Read the model definition and answer for the solid it produces. Units are mm, in the model's axes. Face numbers are marked on the shaded views. A direction names the side the tool comes from. Coordinates: 2 decimals unless noted, no trailing zeros. Write each loop counter-clockwise with the first axis right and the second up, starting at its lowest first coordinate (ties: lowest second). Pieces come first, ordered by that corner, then holes. Notation, with made-up numbers: (48.25, 45.25) -> (81.25, 45.25) arc R31 cw to (81.25, 70.25) -> close; hole circle Ø5 at (73, 83). An arc over 180 degrees is marked (long way). Answer as a JSON object with one key per item and string values. Group by question number.
(1) Find section A-A (z = 28.5). Give the vertices of the cut face in (x, y), then the cut area to 3 significant figures.
(2) Straight lines are drawn through the part: L1, parallel to Z at x = -12, y = -4; L2, parallel to Z at x = 17, y = -2.25; L3, parallel to X at y = 4.75, z = 33. For each, find the intervals that lie inside material, in ascending order.
(3) Find section C-C (x = -38). Give the vertices of the cut face in (y, z), then the cut area to 3 significant figures.
(4) Find section B-B (z = 6.5). Give the vertices of the cut face in (x, y).
(5) Which of the six approach directions +Z, -Z, +X, -X, +Y, -Y give full straight-line access (tool end or side, diameter ignored) to the marked faces 1 and 2?
(6) For a pull along X with two mould halves and no side action, classify the marked faces 3, 4, 5 and 6 as +X half, -X half, draft (parallel to the pull), parting line (faces both ways), or undercut.
(7) Flat-ended cylindrical pins translate along their axes: P1, Ø4, axis at x = -156.5, y = -1.5, coming from the +Z side; P2, Ø6, axis at y = 3.5, z = 30, coming from the -X side; P3, Ø6, axis at y = -6.5, z = 22, coming from the +X side. Find the tip coordinate at first contact, or state that the pin passes through.
(8) Find section D-D (y = -2.25). Give the vertices of the cut face in (x, z).
from build123d import *

# Parameters (mm, degrees)
F1_DEPTH = 35
F3_DEPTH = 10
F5_DEPTH = 12
F6_DEPTH = 12


with BuildPart() as f1:
    # F0 (on Top) → F1 (new body)
    with BuildSketch(Plane.XY):
        with BuildLine():
            Line((-62.8165142711, -9.8129920568), (57.1834857289, -9.8129920568))
            Line((57.1834857289, -9.8129920568), (92.1834857289, -4.8627543336))
            Line((92.1834857289, -4.8627543336), (92.8836937573, -4.7637201565))
            ThreePointArc((92.8836937573, -4.7637201565), (95.958471831, -3.0916320079), (97.1834857289, 0.1870079432))
            ThreePointArc((97.1834857289, 0.1870079432), (95.958471831, 3.4656478942), (92.8836937573, 5.1377360428))
            Line((92.8836937573, 5.1377360428), (57.1834857289, 10.1870079432))
            Line((57.1834857289, 10.1870079432), (-62.8165142711, 10.1870079432))
            Line((-62.8165142711, 10.1870079432), (-162.8165142711, 5.1870079432))
            ThreePointArc((-162.8165142711, 5.1870079432), (-167.8165142711, 0.1870079432), (-162.8165142711, -4.8129920568))
            Line((-162.8165142711, -4.8129920568), (-62.8165142711, -9.8129920568))
        make_face()
    extrude(amount=F1_DEPTH)

    # F2 (on face) → F3 (join)
    with BuildSketch(Plane.XY.offset(35)):
        with BuildLine():
            Line((57.1834857289, 10.1870079432), (27.1834857289, 10.1870079432))
            Line((27.1834857289, 10.1870079432), (27.1834857289, -9.8129920568))
            Line((27.1834857289, -9.8129920568), (57.1834857289, -9.8129920568))
            Line((57.1834857289, -9.8129920568), (92.8836937573, -4.7637201565))
            ThreePointArc((92.8836937573, -4.7637201565), (97.1834857289, 0.1870079432), (92.8836937573, 5.1377360428))
            Line((92.8836937573, 5.1377360428), (57.1834857289, 10.1870079432))
        make_face()
    extrude(amount=F3_DEPTH)

    # F4 (on face) → F5 (cut)
    with BuildSketch(Plane.XY.offset(35)):
        Polygon((2.1834857289, -9.8129920568), (2.1834857289, 10.1870079432), (-62.8165142711, 10.1870079432), (-67.8165142711, 9.9370079432), (-67.8165142711, -9.5629920568), (-62.8165142711, -9.8129920568), align=None)
    extrude(amount=-F5_DEPTH, mode=Mode.SUBTRACT)

    # F4 (on face) → F6 (cut)
    with BuildSketch(Plane.XY.offset(35)):
        Polygon((-102.8165142711, -7.8129920568), (-102.8165142711, 8.1870079432), (-137.8165142711, 6.4370079432), (-137.8165142711, -6.0629920568), align=None)
    extrude(amount=-F6_DEPTH, mode=Mode.SUBTRACT)


solid = f1.part
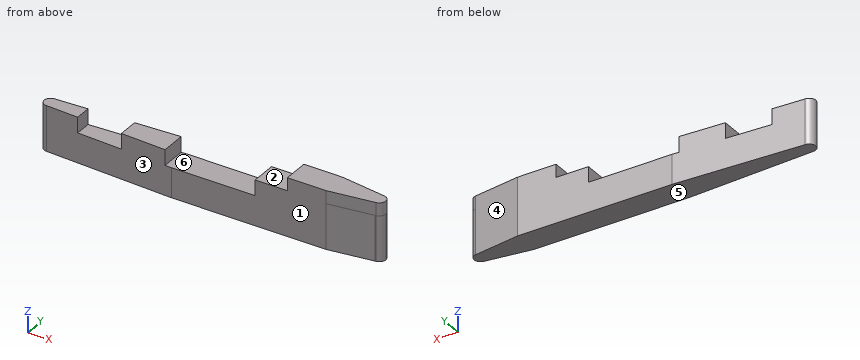
Results below:
{
 "1": {"outline": "(-162.82, -4.81) -> (-137.82, -6.06) -> (-137.82, 6.44) -> (-162.82, 5.19) arc R5 ccw to start; (-102.82, -7.81) -> (-67.82, -9.56) -> (-67.82, 9.94) -> (-102.82, 8.19) -> close; (2.18, -9.81) -> (57.18, -9.81) -> (92.88, -4.76) arc R5 ccw to (92.88, 5.14) -> (57.18, 10.19) -> (2.18, 10.19) -> close", "area": "2,610 mm2"},
 "2": {"L1": "z = 0 to 23", "L2": "z = 0 to 35", "L3": "x = -164.86 to -137.82, -102.82 to -67.82, 2.18 to 94.23"},
 "3": {"outline": "(-9.81, 0) -> (10.19, 0) -> (10.19, 23) -> (-9.81, 23) -> close", "area": "460 mm2"},
 "4": {"outline": "(-162.82, -4.81) -> (-62.82, -9.81) -> (57.18, -9.81) -> (92.88, -4.76) arc R5 ccw to (92.88, 5.14) -> (57.18, 10.19) -> (-62.82, 10.19) -> (-162.82, 5.19) arc R5 ccw to start"},
 "5": {"face 1": "+Z, -Z, +X, -X, -Y", "face 2": "+Z, -X, +Y, -Y"},
 "6": {"face 3": "-X half", "face 4": "+X half", "face 5": "draft", "face 6": "undercut"},
 "7": {"P1": "stops at z = 35", "P2": "stops at x = -167.81", "P3": "stops at x = 95.56"},
 "8": {"outline": "(-167.18, 0) -> (96.55, 0) -> (96.55, 45) -> (27.18, 45) -> (27.18, 35) -> (2.18, 35) -> (2.18, 23) -> (-67.82, 23) -> (-67.82, 35) -> (-102.82, 35) -> (-102.82, 23) -> (-137.82, 23) -> (-137.82, 35) -> (-167.18, 35) -> close"}
}
